Design review of the part built by this model. Coordinates are the model's own, in mm. A direction names the side the tool comes from. Give positions to 0.01 mm unless a question says otherwise; leave off trailing zeros. Write each loop counter-clockwise with the first axis right and the second up, starting at its lowest first coordinate (ties: lowest second). Pieces come first, ordered by that corner, then holes. Notation, with made-up numbers: (-20.75, -0.75) -> (-0.75, -0.75) arc R16 cw to (-0.75, 6.25) -> close; hole circle Ø11 at (-0.5, 7.25). An arc over 180 degrees is marked (long way). Use CSV: the item, a comma, the result in double quotes.
```python
from build123d import *

# Parameters (mm, degrees)
CROQUIS1_R              = 40.5
CROQUIS1_R_2            = 35.5
SALIENTE_EXTRUIR1_DEPTH = 9
CROQUIS2_R              = 2.429274189
SALIENTE_EXTRUIR2_DEPTH = 5
REDONDEO1_R             = 10


with BuildPart() as part:
    # Croquis1 → Saliente-Extruir1 (new body, symmetric)
    with BuildSketch(Plane(origin=(0, 0, 0), x_dir=(1, 0, 0), z_dir=(0, 1, 0))):
        Circle(CROQUIS1_R)
        Circle(CROQUIS1_R_2, mode=Mode.SUBTRACT)
    extrude(amount=SALIENTE_EXTRUIR1_DEPTH, both=True)

    # Croquis2 → Saliente-Extruir2 (add)
    with BuildSketch(Plane.XZ.offset(9)):
        with BuildLine():
            Line((-15, 37.619808612), (-15, 57.619808612))
            Line((-15, 57.619808612), (15, 57.619808612))
            Line((15, 57.619808612), (15, 37.619808612))
            ThreePointArc((15, 37.619808612), (0, 40.5), (-15, 37.619808612))
        make_face()
        with Locations((-9, 47.619808612)):
            Circle(CROQUIS2_R, mode=Mode.SUBTRACT)
        with Locations((9, 47.619808612)):
            Circle(CROQUIS2_R, mode=Mode.SUBTRACT)
    extrude(amount=-SALIENTE_EXTRUIR2_DEPTH)

    # Redondeo1
    redondeo1_edges = [part.edges().sort_by_distance(p)[0] for p in [
        (15, -6.5, 37.619808612),
        (-15, -6.5, 37.619808612),
        (-15, -6.5, 57.619808612),
        (15, -6.5, 57.619808612),
    ]]
    fillet(redondeo1_edges, radius=REDONDEO1_R)


solid = part.part
```
(1) Clearance check with flat-ended pins moving along their axes: pin 1 (4 mm diameter, centred on x = -9, z = 47.62, fed in from -Y); pin 2 (6.5 mm diameter, centred on x = 9, z = 47.62, fed in from +Y); pin 3 (1 mm diameter, centred on x = 27, y = 6, fed in from +Z); pin 4 (1.5 mm diameter, centred on x = 3.5, y = 5.5, fed in from -Z). State where each tip first meets the part, or that it passes through.
Established:
pin 1,"passes through"
pin 2,"stops at y = -4"
pin 3,"stops at z = 30.63"
pin 4,"stops at z = -40.41"
(2) Take a section at C-C (y = -5.5). Write out the cut boundary in (x, z).
Established:
outline,"(-20.05, 35.19) arc R40.5 ccw (long way) to (20.05, 35.19) arc R10 cw to (15, 43.88) -> (15, 47.62) arc R10 ccw to (5, 57.62) -> (-5, 57.62) arc R10 ccw to (-15, 47.62) -> (-15, 43.88) arc R10 cw to start; hole circle Ø71 at (0, 0); hole circle Ø4.86 at (-9, 47.62); hole circle Ø4.86 at (9, 47.62)"
(3) Take a section at A-A (x = -22). Write out the cut boundary in (y, z), then the cut area to 3 significant figures.
Established:
outline,"(-9, -34) -> (9, -34) -> (9, -27.86) -> (-9, -27.86) -> close; (-9, 27.86) -> (9, 27.86) -> (9, 34) -> (-9, 34) -> close"
area,"221 mm2"
(4) Take a section at B-B (z = -9.5). Write out the cut boundary in (x, y), then the cut area to 3 significant figures.
Established:
outline,"(-39.37, -9) -> (-34.21, -9) -> (-34.21, 9) -> (-39.37, 9) -> close; (34.21, -9) -> (39.37, -9) -> (39.37, 9) -> (34.21, 9) -> close"
area,"186 mm2"
(5) Mouldability with a two-part tool opening along X and no side actions: class faces 4 (the face through (-5.272, 0.126, -40.155)), 5 (the face through (0, -4, 47)), 6 (the face through (8.684, -6.535, 50.028)) as +X half, -X half, draft (parallel to the pull), parting line (faces both ways), or undercut.
Established:
face 4,"parting line"
face 5,"draft"
face 6,"undercut"
(6) Tool access review of faces 1 (the face through (-15, -7, 46)), 2 (the face through (-12, -9, 34)), 3 (the face through (15, -7, 46)): name each direction out of +Z, -Z, +X, -X, +Y, -Y from which nothing blocks a thin tool from reaching the whole face with its end or side.
Established:
face 1,"+Z, -X, +Y, -Y"
face 2,"+Z, -Z, +X, -X, -Y"
face 3,"+Z, +X, +Y, -Y"
(7) For line 1 along Z through (x, y) = (-9, -6.9); line 2 along Z through (x, y) = (0, 3.5); line 3 along Z through (x, y) = (-1, -5.75), list the stretches that pass through material, from the lowest coordinate up. Write a range as [from, to].
Established:
line 1,"z = [-39.49, -34.34], [34.34, 45.19], [50.05, 56.78]"
line 2,"z = [-40.5, -35.5], [35.5, 40.5]"
line 3,"z = [-40.49, -35.49], [35.49, 57.62]"
(8) Take a section at D-D (x = 9). Write out the cut boundary in (y, z).
Established:
outline,"(-9, -39.49) -> (9, -39.49) -> (9, -34.34) -> (-9, -34.34) -> close; (-9, 34.34) -> (9, 34.34) -> (9, 39.49) -> (-4, 39.49) -> (-4, 45.19) -> (-9, 45.19) -> close; (-9, 50.05) -> (-4, 50.05) -> (-4, 56.78) -> (-9, 56.78) -> close"
